from build123d import *

# Parameters (mm, degrees)
SKETCH006_W     = 9.5
SKETCH006_H     = 11.1
PAD004_DEPTH    = 6.9
PAD005_DEPTH    = 0.15
POCKET002_DEPTH = 0.25
SKETCH009_R     = 0.8
PAD006_DEPTH    = 0.4
FILLET003_R     = 0.2
SKETCH010_W     = 1
SKETCH010_H     = 0.6
PAD007_DEPTH    = 0.25
FILLET004_R     = 0.24
SKETCH011_W     = 0.75
SKETCH011_H     = 0.5
POCKET003_DEPTH = 9.5
FILLET005_R     = 0.5
POCKET004_DEPTH = 6.25
FILLET006_R     = 0.5
SKETCH013_W     = 3
SKETCH013_H     = 0.65
POCKET005_DEPTH = 0.2


with BuildPart() as part:
    # Sketch006 → Pad004 (new body)
    with BuildSketch(Plane.XZ):
        with Locations((0, -0.7)):
            Rectangle(SKETCH006_W, SKETCH006_H)
    extrude(amount=-PAD004_DEPTH)

    # Sketch007 (on Face6 of Pad004) → Pad005 (join)
    with BuildSketch(Plane(origin=(0, 6.9, 0), x_dir=(1, 0, 0), z_dir=(0, 1, 0))):
        with BuildLine():
            Line((-4.05, 2), (-4.05, -2))
            ThreePointArc((-4.05, -2), (-3.903553, -2.353553), (-3.55, -2.5))
            Line((-3.55, -2.5), (3.55, -2.5))
            ThreePointArc((3.55, -2.5), (3.903553, -2.353553), (4.05, -2))
            Line((4.05, -2), (4.05, 2))
            ThreePointArc((4.05, 2), (3.903553, 2.353553), (3.55, 2.5))
            Line((3.55, 2.5), (-3.55, 2.5))
            ThreePointArc((-3.55, 2.5), (-3.903553, 2.353553), (-4.05, 2))
        make_face()
    extrude(amount=PAD005_DEPTH)

    # Sketch008 (on Face5 of Pad005) → Pocket002 (cut)
    with BuildSketch(Plane(origin=(0, 6.9, 0), x_dir=(1, 0, 0), z_dir=(0, 1, 0))):
        with BuildLine():
            Line((-3.8, -2.7), (-4.75, -2.7))
            Line((-4.75, -2.7), (-4.75, -4.85))
            Line((-4.75, -4.85), (-2.85, -4.85))
            Line((-2.85, -4.85), (-2.85, -3.65))
            ThreePointArc((-2.85, -3.65), (-3.128249, -2.978249), (-3.8, -2.7))
        make_face()
        with BuildLine():
            Line((3.8, 4.6), (4.75, 4.6))
            Line((4.75, 4.6), (4.75, 2.7))
            Line((4.75, 2.7), (3.8, 2.7))
            ThreePointArc((3.8, 4.6), (2.85, 3.65), (3.8, 2.7))
        make_face()
    extrude(amount=-POCKET002_DEPTH, mode=Mode.SUBTRACT)

    # Sketch009 (on Face22 of Pocket002) → Pad006 (join)
    with BuildSketch(Plane(origin=(0, 6.65, 0), x_dir=(1, 0, 0), z_dir=(0, 1, 0))):
        with Locations((3.8, 3.65)):
            Circle(SKETCH009_R)
        with Locations((-3.8, -3.65)):
            Circle(SKETCH009_R)
    extrude(amount=PAD006_DEPTH)

    # Fillet003
    fillet003_edges = [part.edges().sort_by_distance(p)[0] for p in [
        (3, 7.05, -3.65),
        (-4.6, 7.05, 3.65),
    ]]
    fillet(fillet003_edges, radius=FILLET003_R)

    # Sketch010 (on Face12 of Fillet003) → Pad007 (join)
    with BuildSketch(Plane(origin=(0, 0, -6.25), x_dir=(1, 0, 0), z_dir=(0, 0, -1))):
        with Locations((-4.25, -0.8)):
            Rectangle(SKETCH010_W, SKETCH010_H)
        with Locations((-4.25, -6.55)):
            Rectangle(SKETCH010_W, SKETCH010_H)
        with Locations((4.25, -0.8)):
            Rectangle(SKETCH010_W, SKETCH010_H)
        with Locations((4.25, -6.55)):
            Rectangle(SKETCH010_W, SKETCH010_H)
    extrude(amount=PAD007_DEPTH)

    # Fillet004
    fillet004_edges = [part.edges().sort_by_distance(p)[0] for p in [
        (-3.75, 0.8, -6.5),
        (-4.75, 0.8, -6.5),
        (3.75, 0.8, -6.5),
        (4.75, 0.8, -6.5),
        (4.75, 6.55, -6.5),
        (3.75, 6.55, -6.5),
        (-3.75, 6.55, -6.5),
        (-4.75, 6.55, -6.5),
    ]]
    fillet(fillet004_edges, radius=FILLET004_R)

    # Sketch011 (on Face16 of Fillet004) → Pocket003 (cut)
    with BuildSketch(Plane(origin=(4.75, 0, 0), x_dir=(0, 0, 1), z_dir=(1, 0, 0))):
        with Locations((-5.875, -0.25)):
            Rectangle(SKETCH011_W, SKETCH011_H)
    extrude(amount=-POCKET003_DEPTH, mode=Mode.SUBTRACT)

    # Fillet005
    fillet005_edges = [part.edges().sort_by_distance(p)[0] for p in [
        (-4.75, 3.675, -6.25),
        (4.75, 3.675, -6.25),
    ]]
    fillet(fillet005_edges, radius=FILLET005_R)

    # Sketch012 (on Face25 of Fillet005) → Pocket004 (cut)
    with BuildSketch(Plane.XZ):
        with BuildLine():
            Line((3.75, 4.85), (3.75, 5.85))
            Line((3.75, 5.85), (5.75, 5.85))
            Line((5.75, 5.85), (5.75, 3.85))
            Line((5.75, 3.85), (4.75, 3.85))
            ThreePointArc((4.75, 3.85), (4.457107, 4.557107), (3.75, 4.85))
        make_face()
        with BuildLine():
            ThreePointArc((-3.75, 4.85), (-4.457107, 4.557107), (-4.75, 3.85))
            Line((-5.75, 3.85), (-4.75, 3.85))
            Line((-5.75, 5.85), (-5.75, 3.85))
            Line((-3.75, 5.85), (-5.75, 5.85))
            Line((-3.75, 4.85), (-3.75, 5.85))
        make_face()
    extrude(amount=-POCKET004_DEPTH, mode=Mode.SUBTRACT)

    # Fillet006
    fillet006_edges = [part.edges().sort_by_distance(p)[0] for p in [
        (4.75, 6.575, 4.85),
        (-4.75, 6.45, 4.85),
    ]]
    fillet(fillet006_edges, radius=FILLET006_R)

    # Sketch013 (on Face17 of Fillet006) → Pocket005 (cut)
    with BuildSketch(Plane(origin=(0, 0, 4.85), x_dir=(-1, 0, 0), z_dir=(0, 0, 1))):
        with Locations((0, -6.575)):
            Rectangle(SKETCH013_W, SKETCH013_H)
    extrude(amount=-POCKET005_DEPTH, mode=Mode.SUBTRACT)


solid = part.part
The listing builds one solid part. Answer for the finished solid, in the listing's coordinates (mm). A direction names the side the tool comes from. Round coordinates to 2 decimals unless told otherwise and drop trailing zeros. Order: outer loops, then holes, each group sorted by start corner. A loop starts at its lowest first (then second) coordinate and runs counter-clockwise, first axis right, second up. Notation, with made-up numbers: (73.25, 65) -> (85.25, 65) arc R26 ccw to (85.25, 90) -> close; hole circle Ø6 at (-0.75, 89.5). An arc over 180 degrees is marked (long way). One line per item, written item: value.
Item 1: Straight lines are drawn through the part: L1, parallel to Z at x = 1.5, y = 3.25; L2, parallel to Y at x = 0.5, z = -4.5; L3, parallel to X at y = 4.5, z = 4. For each, find the intervals that lie inside material, in ascending order.
Taken from the geometry:
L1: z = -6.25 to 4.85
L2: y = 0 to 6.9
L3: x = -4.74 to 4.74
Item 2: Find section A-A, the plane x = 1.75. Give the vertices of the cut face in (y, z).
Taken from the geometry:
outline: (0, -5.5) -> (0.5, -5.5) -> (0.5, -6.25) -> (6.9, -6.25) -> (6.9, -2.5) -> (7.05, -2.5) -> (7.05, 2.5) -> (6.9, 2.5) -> (6.9, 4.85) -> (0, 4.85) -> close
Item 3: For faces 1 (the flat face through (0, 0.5, -6)), 2 (the cylindrical face through (4.465, 3.081, 4.549)), 3 (the flat face through (0, 6.9, -3)), 4 (the cylindrical face through (-4.449, 3.081, 4.565)), determine the directions among +Z, -Z, +X, -X, +Y, -Y from which every point of the face is accessible in a straight line to the end or side of a thin tool.
Taken from the geometry:
face 1: -Z, +X, -X, -Y
face 2: +Z, +X, -Y
face 3: +Y
face 4: +Z, -X, -Y
Item 4: Given P1, Ø3, axis at x = 3.5, z = -5, coming from the -Y side; P2, Ø0.6, axis at x = 1, y = 0, coming from the -Z side; P3, Ø1.5, axis at x = 1.5, y = 4, coming from the -Z side; P4, Ø0.6, axis at x = -4, z = -6, coming from the +Y side, each flat-ended and moving along its own axis, determine where each tip first touches the part or whether it passes through.
Taken from the geometry:
P1: stops at y = 0
P2: stops at z = -5.5
P3: stops at z = -6.25
P4: stops at y = 6.9
Item 5: Find section D-D, the plane x = -1.25. Give the vertices of the cut face in (y, z).
Taken from the geometry:
outline: (0, -5.5) -> (0.5, -5.5) -> (0.5, -6.25) -> (6.9, -6.25) -> (6.9, -2.5) -> (7.05, -2.5) -> (7.05, 2.5) -> (6.9, 2.5) -> (6.9, 4.65) -> (6.25, 4.65) -> (6.25, 4.85) -> (0, 4.85) -> close
Item 6: Find section B-B, the plane z = -3.65. Give the vertices of the cut face in (x, y), then the cut area to 3 significant figures.
Taken from the geometry:
outline: (-4.75, 0) -> (4.75, 0) -> (4.75, 6.65) -> (4.6, 6.65) -> (4.6, 6.85) arc R0.2 ccw to (4.4, 7.05) -> (3.2, 7.05) arc R0.2 ccw to (3, 6.85) -> (3, 6.65) -> (2.85, 6.65) -> (2.85, 6.9) -> (-4.75, 6.9) -> close
area: 65.7 mm2
Item 7: Find section C-C, the plane y = 3. Give the vertices of the cut face in (x, z), then the cut area to 3 significant figures.
Taken from the geometry:
outline: (-4.75, -5.75) arc R0.5 ccw to (-4.25, -6.25) -> (4.25, -6.25) arc R0.5 ccw to (4.75, -5.75) -> (4.75, 3.85) arc R1 ccw to (3.75, 4.85) -> (-3.75, 4.85) arc R1 ccw to (-4.75, 3.85) -> close
area: 105 mm2
